For this review, take the finished solid that the model builds, in its own axes (mm). Face numbers are marked on the shaded views. Coordinates: 2 decimals unless noted, no trailing zeros. Write each loop counter-clockwise with the first axis right and the second up, starting at its lowest first coordinate (ties: lowest second). Pieces come first, ordered by that corner, then holes.
1) We need section A-A on z = 1.75. Write out the cut boundary in (x, y), then the cut area to 3 significant figures.
2) We need section C-C on x = -101.75. Give the number of separate pieces and of enclosed holes in the cut face, then the cut area to 3 significant figures.
3) We need section D-D on x = -97.25. Write out the cut boundary in (y, z), then the cut area to 3 significant figures.
4) Mouldability with a two-part tool opening along Y and no side actions: class the marked faces 1, 2 and 3 as pulls with the +Y half, pulls with the -Y half, needs draft (parallel to the pull), parting line crosses it, or undercut.
5) We need section B-B on x = -107. Write out the cut boundary in (y, z).
6) To check wall thickness, follow line 1 along Y through (x, z) = (-101, 8); line 2 along X through (y, z) = (47.25, 4); line 3 along X through (y, z) = (44.5, 4.5). State the ranges of each line that lie inside material, in increasing order.
7) Insertion check: P1, Ø1, axis at y = 39, z = 4, coming from the +X side; P2, Ø1.5, axis at y = 40.5, z = 8, coming from the +X side. Each pin has a flat end and moves straight along its axis. Give the tip position at first contact, or say it passes through.
from build123d import *

# Parameters (mm, degrees)
SKETCH1_R                   = 5.95
BOSS_EXTRUDE2_DEPTH         = 10
SKETCH12_R                  = 0.95
CUT_EXTRUDE3_DEPTH          = 10
F_37_0_104_DIAMETER_HOLE1_D = 2.6416


with BuildPart() as part:
    # Sketch1 → Boss-Extrude2 (new body)
    with BuildSketch(Plane.XY):
        with Locations((-101.724686529, 42.083000392)):
            Circle(SKETCH1_R)
    extrude(amount=BOSS_EXTRUDE2_DEPTH)

    # Sketch12 → Cut-Extrude3 (cut)
    with BuildSketch(Plane.XY.offset(10)):
        with Locations((-101.724686529, 42.083000392)):
            Circle(SKETCH12_R)
    extrude(amount=-CUT_EXTRUDE3_DEPTH, mode=Mode.SUBTRACT)

    # #37 (0.104) Diameter Hole1 (through all)
    with Locations(Plane(origin=(-101.228935977, 36.153689185, 4.736849069), x_dir=(-0.996522891944, -0.083319420496, 0), z_dir=(0.083319420496, -0.996522891944, 0))):
        with Locations((0, 0)):
            Hole(F_37_0_104_DIAMETER_HOLE1_D / 2)


solid = part.part
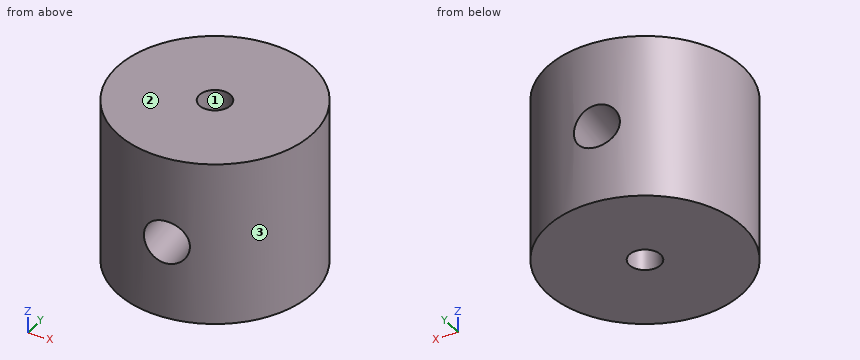
Result:
1. outline: circle Ø11.9 at (-101.72, 42.08); hole circle Ø1.9 at (-101.72, 42.08)
1. area: 108 mm2
2. separate pieces: 4
2. enclosed holes: 0
2. area: 74.3 mm2
3. outline: (38.16, 0) - (46, 0) - (46, 10) - (38.16, 10) - close
3. area: 78.4 mm2
4. face 1: undercut
4. face 2: needs draft
4. face 3: parting line crosses it
5. outline: (39.33, 0) - (44.84, 0) - (44.84, 10) - (39.33, 10) - close
6. line 1: y = 36.18 to 41.47, 42.7 to 47.99
6. line 2: x = -104.68 to -103.26, -101.06 to -98.77
6. line 3: x = -107.16 to -103.23, -100.62 to -96.29
7. P1: stops at x = -96.36
7. P2: stops at x = -95.83
